Could you check a few things on this model? Use its own coordinates, in mm. A direction names the side the tool comes from. Give positions to 0.01 mm unless a question says otherwise; leave off trailing zeros. Loops run counter-clockwise (first coordinate to the right, second up) from the corner with the lowest first, then second, coordinate; pieces in that order, holes last. Notation, with made-up numbers: (88.25, 23.5) -> (124.25, 23.5) arc R29 cw to (124.25, 50.5) -> close; hole circle Ø9 at (71, -22). An arc over 180 degrees is marked (long way). Write item = value, one per line. Start each with the question number.
1) I want a section at C-C (y = 12). List the corners of the cut face in (x, z) for me, and give its area (3 significant figures).
2) I want a section at B-B (x = 71.5). List the corners of the cut face in (y, z) for me, and give its area (3 significant figures).
3) If we mould it in two halves opening along X, with no side actions, what happens to faces 1 (the face through (78.779, -36.254, -9.367)), 2 (the face through (28, 55, 0)), 3 (the face through (-3.47, 15.62, 15.51)), 4 (the face through (-32, 0, 25))? For each: +X half, -X half, draft (parallel to the pull), parting line (faces both ways), or undercut.
4) On a 3-axis mill with a long thin cutter (end or side, diameter ignored), from which of +Z, -Z, +X, -X, +Y, -Y can I reach the whole of each face in a straight line? I mean faces 5 (the face through (-63, 1, 0)), 6 (the face through (-55.417, -96.209, 1.952)), 7 (the face through (15.69, 27.89, 25.14)). Say none if no direction works.
5) I need wall thicknesses on probe 1 along Y at (x, z) = (0, -6.75); probe 2 along X at (y, z) = (36.5, -2); probe 3 along Y at (x, z) = (-26, 1.5). Which ranges of each line are inside material? Lowest first, please. Write a range as from..to.
6) I want a section at A-A (y = -40). Count the separate pieces of the cut face and the enclosed holes in it, and give its area (3 significant figures).
7) I'm going to push flat-ended pins straight in: pin 1 Ø3 at (x, z) = (30.5, -11) entering from -Y; pin 2 Ø3 at (x, z) = (64, 9) entering from +Y; pin 3 Ø21 at (x, z) = (60.5, 12) entering from -Y. Where does each tip first touch, or does it pass through?
Solid Edge part; units mm, degrees
sketch "Sketch1" plane through (0, 0, 0) normal (0, 0, 1) x (1, 0, 0)
  circle A0 centre (0, 0) radius 101.5
extrude "Protrusion1" add sketch "Sketch1" against normal blind 19
sketch "Sketch2" plane through (0, 0, 0) normal (0, 0, 1) x (1, 0, 0)
  circle A0 centre (0, 0) radius 32
extrude "ExtrudedProtrusion_2" add sketch "Sketch2" along normal blind 51
sketch "Sketch3" plane through (0, 0, 0) normal (0, 0, 1) x (1, 0, 0)
  circle A0 centre (0, 0) radius 16
extrude "ExtrudedCutout_1" cut sketch "Sketch3" along normal blind 51
sketch "Sketch4" plane through (0, 0, 0) normal (0, 0, 1) x (1, 0, 0)
  circle A0 centre (0, 0) radius 16
extrude "ExtrudedCutout_2" cut sketch "Sketch4" against normal blind 19
sketch "Sketch5" plane through (0, 0, 0) normal (0, 0, 1) x (1, 0, 0)
  circle A0 centre (0, 86) radius 8
extrude "ExtrudedCutout_3" cut sketch "Sketch5" against normal blind 19
sketch "Sketch6" plane through (0, 0, 0) normal (0, 0, 1) x (1, 0, 0)
  circle A0 centre (74.4782, 43) radius 8
  circle A1 centre (74.4782, -43) radius 8
  circle A2 centre (0, -86) radius 8
  circle A3 centre (-74.4782, -43) radius 8
  circle A4 centre (-74.4782, 43) radius 8
  circle A5 centre (0, 86) radius 8
extrude "ExtrudedCutout_4" cut sketch "Sketch6" against normal blind 19
sketch "Sketch7" plane through (0, 0, 0) normal (0, 0, 1) x (0, 1, 0)
  line L0 (-105.758, 51.8218) -> (-30.8328, 8.5637)
  arc A0 (-30.8328, 8.5637) -> (-22.8328, 22.4201) centre (0, 0) cw
  line L1 (-22.8328, 22.4201) -> (-97.758, 65.6782)
  line L2 (-101.758, 58.75) -> (-97.758, 65.6782)
  line L3 (-101.758, 58.75) -> (-105.758, 51.8218)
  line L4 (105.758, 51.8218) -> (31.1942, 8.7724)
  line L5 (31.1942, 8.7724) -> (30.8328, 8.5637)
  arc A1 (22.8328, 22.4201) -> (30.8328, 8.5637) centre (0, 0) cw
  line L6 (22.8328, 22.4201) -> (97.758, 65.6782)
  line L7 (97.758, 65.6782) -> (105.758, 51.8218)
  line L8 (8, -30.9839) -> (8, -117.5)
  line L9 (0, -117.5) -> (8, -117.5)
  line L10 (0, -117.5) -> (-8, -117.5)
  line L11 (-8, -117.5) -> (-8, -30.9839)
  arc A2 (8, -30.9839) -> (-8, -30.9839) centre (0, 0) cw
extrude "ExtrudedProtrusion_5" add sketch "Sketch7" along normal blind 51
sketch "Sketch8" plane through (0, 0, 0) normal (0, 0, 1) x (0, 1, 0)
  line L0 (-105.758, 51.8218) -> (-30.8328, 8.5637)
  arc A0 (-30.8328, 8.5637) -> (-22.8328, 22.4201) centre (0, 0) cw
  line L1 (-22.8328, 22.4201) -> (-97.758, 65.6782)
  line L2 (-101.758, 58.75) -> (-97.758, 65.6782)
  line L3 (-101.758, 58.75) -> (-105.758, 51.8218)
  line L4 (-8, -117.5) -> (-8, -30.9839)
  line L5 (8, -30.9839) -> (8, -117.5)
  line L6 (0, -117.5) -> (8, -117.5)
  line L7 (0, -117.5) -> (-8, -117.5)
  arc A1 (8, -30.9839) -> (-8, -30.9839) centre (0, 0) cw
  line L8 (105.758, 51.8218) -> (31.1942, 8.7724)
  line L9 (31.1942, 8.7724) -> (30.8328, 8.5637)
  arc A2 (22.8328, 22.4201) -> (30.8328, 8.5637) centre (0, 0) cw
  line L10 (22.8328, 22.4201) -> (97.758, 65.6782)
  line L11 (97.758, 65.6782) -> (105.758, 51.8218)
extrude "ExtrudedProtrusion_6" add sketch "Sketch8" against normal blind 19
sketch "Sketch9" plane through (-30.1928, -68.2954, 16) normal (0.8660254, -0.5, 0) x (0.5, 0.8660254, 0)
  line L0 (-43.2581, 35) -> (43.2581, 35)
  line L1 (43.2581, 35) -> (-43.2581, 4.0795)
  line L2 (-43.2581, 4.0795) -> (-43.2581, 35)
extrude "ExtrudedCutout_5" cut sketch "Sketch9" against normal blind 16
sketch "Sketch10" plane through (-30.1928, -68.2954, 16) normal (0.8660254, -0.5, 0) x (0.5, 0.8660254, 0)
  arc A0 (-43.2581, -35) -> (-47.8653, 2.4329) centre (-43.2581, -16) cw
  line L0 (43.2581, 35) -> (-47.8653, 2.4329)
  line L1 (-43.2581, -35) -> (43.2581, -35)
  line L2 (43.2581, 35) -> (43.2581, -35)
extrude "ExtrudedProtrusion_7" add sketch "Sketch10" against normal blind 16
extrude "Cutout1" [suppressed]
extrude "ExtrudedCutout_7" [suppressed]
sketch "Sketch11" plane through (74.2419, -8, 16) normal (0, -1, 0) x (1, 0, 0)
  line L0 (-43.2581, -35) -> (43.2581, -35)
  line L1 (-43.2581, 35) -> (-43.2581, -35)
  line L2 (-43.2581, 35) -> (43.2601, 4.1696)
  line L3 (43.2601, 4.1696) -> (49.6358, 1.8976)
  arc A0 (49.6358, 1.8976) -> (43.2581, -35) centre (43.2581, -16) cw
extrude "Protrusion2" add sketch "Sketch11" against normal blind 16
sketch "Sketch12" plane through (74.2419, -8, 16) normal (0, -1, 0) x (1, 0, 0)
  line L0 (-43.2581, 35) -> (43.2581, 35)
  line L1 (43.2581, 35) -> (43.2601, 4.1696)
  line L2 (-43.2581, 35) -> (43.2601, 4.1696)
extrude "ExtrudedCutout_8" cut sketch "Sketch12" against normal blind 16
extrude "Cutout2" [suppressed]
sketch "Sketch13" plane through (-30.1928, -68.2954, 16) normal (0.8660254, -0.5, 0) x (0.5, 0.8660254, 0)
  arc A0 (-43.2581, -35) -> (-47.8653, 2.4329) centre (-43.2581, -16) cw
  line L0 (43.2581, 35) -> (-47.8653, 2.4329)
  line L1 (-43.2581, -35) -> (43.2581, -35)
  line L2 (43.2581, 35) -> (43.2581, -35)
extrude "ExtrudedProtrusion_13" add sketch "Sketch13" against normal blind 16.01
sketch "Sketch14" plane through (-30.1928, -68.2954, 16) normal (0.8660254, -0.5, 0) x (0.5, 0.8660254, 0)
  circle A0 centre (-42.9854, -16) radius 6.5
extrude "Cutout3" cut sketch "Sketch14" against normal blind 16
sketch "Sketch15" plane through (-30.1928, 68.2954, 16) normal (0.8660254, 0.5, 0) x (-0.5, 0.8660254, 0)
  line L0 (43.2581, -35) -> (43.2581, 3)
  arc A0 (43.2581, 3) -> (43.2581, -35) centre (43.2581, -16) cw
extrude "ExtrudedProtrusion_14" add sketch "Sketch15" against normal blind 16
sketch "Sketch16" plane through (-30.1928, 68.2954, 16) normal (0.8660254, 0.5, 0) x (-0.5, 0.8660254, 0)
  line L0 (43.2581, 35) -> (-43.2581, 35)
  line L1 (-43.2581, 35) -> (43.2581, 3)
  line L2 (43.2581, 3) -> (43.2581, 35)
extrude "Cutout4" cut sketch "Sketch16" against normal blind 16
Answer list:
q1.outline = (-100.79, -19) -> (-10.58, -19) -> (-10.58, 51) -> (-29.66, 51) -> (-29.66, 0) -> (-100.79, 0) -> close; (10.58, -19) -> (100.79, -19) -> (100.79, 0) -> (29.66, 0) -> (29.66, 51) -> (10.58, 51) -> close
q1.area = 5,370 mm^2
q2.outline = (-72.04, -19) -> (-50.42, -19) -> (-50.42, 0) -> (-72.04, 0) -> close; (-35.58, -19) -> (35.58, -19) -> (35.58, 0) -> (8, 0) -> (8, 36.56) -> (-8, 36.56) -> (-8, 0) -> (-35.58, 0) -> close; (50.42, -19) -> (72.04, -19) -> (72.04, 0) -> (50.42, 0) -> close
q2.area = 2,760 mm^2
q3.face_1 = undercut
q3.face_2 = draft
q3.face_3 = undercut
q3.face_4 = -X half
q4.face_5 = +Z, -X
q4.face_6 = none
q4.face_7 = +Z, +Y
q5.probe_1 = -101.5..-94, -78..-16, 16..78, 94..101.5
q5.probe_2 = -94.71..-79.14, -69.81..69.81, 79.14..94.71
q5.probe_3 = -61.03..-29.01, -18.65..18.65, 29.03..61.03
q6.separate_pieces = 3
q6.enclosed_holes = 0
q6.area = 3,820 mm^2
q7.pin_1 = -97.27
q7.pin_2 = 8
q7.pin_3 = -8
